from build123d import *

# Parameters (mm, degrees)
F0_R     = 3.15
F1_DEPTH = 4.7625


with BuildPart() as f1:
    # F0 (on Front) → F1 (new body)
    with BuildSketch(Plane.XZ):
        with BuildLine():
            Line((-6.671903, -9), (97.890261, -9))
            ThreePointArc((97.890261, -9), (98.40446, -8.857671), (98.772288, -8.471199))
            Line((98.772288, -8.471199), (101.407221, -3.53893))
            ThreePointArc((101.407221, -3.53893), (101.523973, -3.018327), (101.356414, -2.511787))
            Line((101.356414, -2.511787), (44.558999, 82.408944))
            ThreePointArc((44.558999, 82.408944), (44.198978, 82.735027), (43.727779, 82.853))
            Line((43.727779, 82.853), (34.657767, 82.853))
            ThreePointArc((34.657767, 82.853), (34.143569, 82.710671), (33.775741, 82.324199))
            Line((33.775741, 82.324199), (-11.082037, -1.644003))
            ThreePointArc((-11.082037, -1.644003), (-10.960259, -6.570994), (-6.671903, -9))
        make_face()
        Circle(F0_R, mode=Mode.SUBTRACT)
        with Locations((42.768, 24.618)):
            Circle(F0_R, mode=Mode.SUBTRACT)
        with Locations((88.849, 0)):
            Circle(F0_R, mode=Mode.SUBTRACT)
        with Locations((39.454, 73.853)):
            Circle(F0_R, mode=Mode.SUBTRACT)
    extrude(amount=F1_DEPTH)


solid = f1.part
Could you check a few things on this model? Use its own coordinates, in mm. Give positions to 0.01 mm unless a question says otherwise; leave off trailing zeros. Write each loop counter-clockwise with the first axis right and the second up, starting at its lowest first coordinate (ties: lowest second). Pieces come first, ordered by that corner, then holes. Notation, with made-up numbers: (4.25, 52.5) -> (60.25, 52.5) arc R25 cw to (60.25, 81.5) -> close; hole circle Ø3 at (-26, 33.25). An arc over 180 degrees is marked (long way). Answer as CSV lines item,"result". Start each with the question number.
(1) I'm going to push flat-ended pins straight in: pin 1 Ø1 at (x, z) = (15, 3.5) entering from +Y; pin 2 Ø5 at (x, z) = (88.849, 0) entering from +Y; pin 3 Ø2 at (y, z) = (-1, 22.5) entering from +X. Where does each tip first touch, or does it pass through?
(2) Please list where these lines run through material, in increasing order: line 1 (Z direction, x = -0.5, y = -0.9); line 2 (Z direction, x = 39, y = -1.65); line 3 (X direction, y = -0.25, z = 23).
(3) If we mould it in two halves opening along Z, with no side actions, what happens to faces 1 (the face through (11.66, -2.35, 40.93)), 2 (the face through (45, -2, -9)), 3 (the face through (40.91, -2.35, 71.06)), 4 (the face through (44, 0, 17))? For each: +Z half, -Z half, draft (parallel to the pull), parting line (faces both ways), or undercut.
(4) If we section it at C-C, the plane y = -2.4: Write out the boundary of the cut face in (x, z), and give its area (3 significant figures).
(5) If we section it at A-A, the plane z = 0: Write out the boundary of the cut face in (x, y).
(6) If we section it at B-B, the plane x = 0: Write out the boundary of the cut face in (y, z), and give its area (3 significant figures).
(7) If we section it at D-D, the plane x = 50: Write out the boundary of the cut face in (y, z), and give its area (3 significant figures).
Answer list:
1,pin 1,"y = 0"
1,pin 2,"through"
1,pin 3,"x = 85.3"
2,line 1,"-9 to -3.11, 3.11 to 18.16"
2,line 2,"-9 to 70.74, 76.97 to 82.85"
2,line 3,"2.08 to 40.07, 45.47 to 84.29"
3,face 1,"+Z half"
3,face 2,"-Z half"
3,face 3,"undercut"
3,face 4,"draft"
4,outline,"(-11.08, -1.64) arc R5 ccw to (-6.67, -9) -> (97.89, -9) arc R1 ccw to (98.77, -8.47) -> (101.41, -3.54) arc R1 ccw to (101.36, -2.51) -> (44.56, 82.41) arc R1 ccw to (43.73, 82.85) -> (34.66, 82.85) arc R1 ccw to (33.78, 82.32) -> close; hole circle Ø6.3 at (0, 0); hole circle Ø6.3 at (39.45, 73.85); hole circle Ø6.3 at (42.77, 24.62); hole circle Ø6.3 at (88.85, 0)"
4,area,"5,850 mm^2"
5,outline,"(-10.2, -4.76) -> (-3.15, -4.76) -> (-3.15, 0) -> (-10.2, 0) -> close; (3.15, -4.76) -> (85.7, -4.76) -> (85.7, 0) -> (3.15, 0) -> close; (92, -4.76) -> (99.68, -4.76) -> (99.68, 0) -> (92, 0) -> close"
6,outline,"(-4.76, -9) -> (0, -9) -> (0, -3.15) -> (-4.76, -3.15) -> close; (-4.76, 3.15) -> (0, 3.15) -> (0, 19.1) -> (-4.76, 19.1) -> close"
6,area,"104 mm^2"
7,outline,"(-4.76, -9) -> (0, -9) -> (0, 74.27) -> (-4.76, 74.27) -> close"
7,area,"397 mm^2"
